The model under review builds one solid part; all positions refer to its coordinate system, in mm. Face numbers are marked on the shaded views. A direction names the side the tool comes from. Give positions to 0.01 mm unless a question says otherwise; leave off trailing zeros. Order: outer loops, then holes, each group sorted by start corner. A loop starts at its lowest first (then second) coordinate and runs counter-clockwise, first axis right, second up.
```python
from build123d import *

# Parameters (mm, degrees)
SKETCH_1_R          = 7.5
EXTRUDE_1_DEPTH     = 12.6
SKETCH_2_W          = 11.291748881
SKETCH_2_H          = 5
EXTRUDE_2_DEPTH     = 32.6
SKETCH_3_R          = 1.5
CUT_EXTRUDE_1_DEPTH = 45.373528145
FILLET_1_R          = 3
SKETCH_4_W          = 3
SKETCH_4_H          = 10
EXTRUDE_3_DEPTH     = 20
SKETCH_5_R          = 1.3
CUT_EXTRUDE_2_DEPTH = 46.967488511
SKETCH_6_W          = 35.293936169
SKETCH_6_H          = 34.958158763
CUT_EXTRUDE_3_DEPTH = 46.967488511
EXTRUDE_4_OUTLINE_R = 1.55
EXTRUDE_4_DEPTH     = 3
SKETCH_8_R          = 1.900956558
CUT_EXTRUDE_4_DEPTH = 46.967488511
SKETCH_9_R          = 3
CUT_EXTRUDE_5_DEPTH = 3


# Read off the part's stored shape, not the designer's step: 凸台-拉伸4
with BuildPart() as part:
    # 草图1 → 凸台-拉伸1 (new body)
    with BuildSketch(Plane.XY):
        with BuildLine():
            Line((-10.956194261, 6.017624724), (-22.5, -15))
            Line((-22.5, -15), (-22.5, -20))
            Line((-22.5, -20), (22.5, -20))
            Line((22.5, -20), (22.5, -15))
            Line((22.5, -15), (10.956194261, 6.017624724))
            ThreePointArc((10.956194261, 6.017624724), (0, 12.5), (-10.956194261, 6.017624724))
        make_face()
        Circle(SKETCH_1_R, mode=Mode.SUBTRACT)
    extrude(amount=EXTRUDE_1_DEPTH)

    # 草图2 → 凸台-拉伸2 (add)
    with BuildSketch(Plane.XY):
        with Locations((-16.854125559, -17.5)):
            Rectangle(SKETCH_2_W, SKETCH_2_H)
        with Locations((16.854125559, -17.5)):
            Rectangle(SKETCH_2_W, SKETCH_2_H)
    extrude(amount=EXTRUDE_2_DEPTH)

    # 草图3 → 切除-拉伸1 (cut, through all)
    with BuildSketch(Plane(origin=(0, 0, 0), x_dir=(1, 0, 0), z_dir=(0, 1, 0))):
        with Locations(Location((-17.5, -26.3, 0), (0, 0, 270))):
            Circle(SKETCH_3_R)
        with Locations((17.5, -26.3)):
            Circle(SKETCH_3_R)
    extrude(amount=-CUT_EXTRUDE_1_DEPTH, mode=Mode.SUBTRACT)

    # 圆角1
    fillet_1_edges = [part.edges().sort_by_distance(p)[0] for p in [
        (-22.5, -17.5, 32.6),
        (-11.208251119, -17.5, 32.6),
        (11.208251119, -17.5, 32.6),
    ]]
    fillet(fillet_1_edges, radius=FILLET_1_R)

    # 草图4 → 凸台-拉伸3 (add, through all)
    with BuildSketch(Plane(origin=(0, 0, 0), x_dir=(1, 0, 0), z_dir=(0, 1, 0))):
        with Locations((24, -27.6)):
            Rectangle(SKETCH_4_W, SKETCH_4_H)
    extrude(amount=-EXTRUDE_3_DEPTH)

    # 草图5 → 切除-拉伸2 (cut, through all)
    with BuildSketch(Plane(origin=(0, 0, 0), x_dir=(0, 0, -1), z_dir=(1, 0, 0))):
        with Locations(Location((-27.6, -3, 0), (0, 0, 180))):
            Circle(SKETCH_5_R)
        with Locations(Location((-27.6, -12.5, 0), (0, 0, 180))):
            Circle(SKETCH_5_R)
    extrude(amount=CUT_EXTRUDE_2_DEPTH, mode=Mode.SUBTRACT)

    # 草图6 → 切除-拉伸3 (cut, through all)
    with BuildSketch(Plane(origin=(0, 0, 0), x_dir=(0, 0, -1), z_dir=(1, 0, 0))):
        with Locations((-16.337308601, -3.7126914)):
            Rectangle(SKETCH_6_W, SKETCH_6_H)
    extrude(amount=-CUT_EXTRUDE_3_DEPTH, mode=Mode.SUBTRACT)

    # 凸台-拉伸4 outline → 凸台-拉伸4 (add)
    with BuildSketch(Plane(origin=(0, 0, 0), x_dir=(0, 0, -1), z_dir=(1, 0, 0))):
        with BuildLine():
            Line((-9.3, 15.5), (-9.3, 9.152926334))
            Line((-9.3, 9.152926334), (-3.3, 9.152926334))
            Line((-3.3, 9.152926334), (-3.3, 15.5))
            ThreePointArc((-3.3, 15.5), (-6.3, 18.5), (-9.3, 15.5))
        make_face()
        with Locations((-6.3, 15.5)):
            Circle(EXTRUDE_4_OUTLINE_R, mode=Mode.SUBTRACT)
    extrude(amount=EXTRUDE_4_DEPTH)

    # 草图8 → 切除-拉伸4 (cut, through all)
    with BuildSketch(Plane(origin=(0, 0, 0), x_dir=(0, 0, -1), z_dir=(1, 0, 0))):
        with Locations(Location((-6.3, -12.5, 0), (0, 0, 90))):
            Circle(SKETCH_8_R)
    extrude(amount=CUT_EXTRUDE_4_DEPTH, mode=Mode.SUBTRACT)

    # 草图9 → 切除-拉伸5 (cut)
    with BuildSketch(Plane(origin=(22.5, 0, 0), x_dir=(0, 0, -1), z_dir=(1, 0, 0))):
        with Locations((-6.3, -12.5)):
            Circle(SKETCH_9_R)
    extrude(amount=-CUT_EXTRUDE_5_DEPTH, mode=Mode.SUBTRACT)


solid = part.part
```
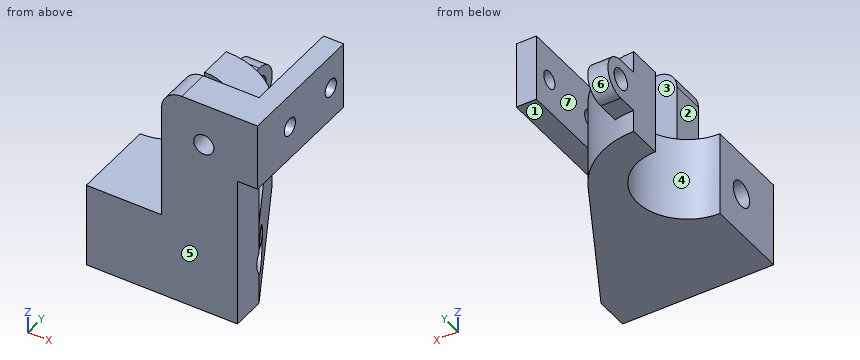
1. Take a section at A-A (x = 17.5). Write out the cut boundary in (y, z), and give its area (3 significant figures).
2. For the marked faces 1, 2 and 3, list the 3-axis set-ups (+Z, -Z, +X, -X, +Y, -Y) from which the entire face can be reached by the end or side of a thin tool; tool diameter is ignored.
3. Insertion check: pin 1 (9.5 mm diameter, centred on y = -12.5, z = 6.3, fed in from +X); pin 2 (3.5 mm diameter, centred on x = 18.5, z = 23, fed in from +Y); pin 3 (1.5 mm diameter, centred on x = 1.5, y = 13.5, fed in from +Z); pin 4 (3 mm diameter, centred on y = -12.5, z = 6.3, fed in from +X). Each pin has a flat end and moves straight along its axis. Give the tip position at first contact, or say it passes through.
4. Take a section at C-C (z = 24). Write out the cut boundary in (x, y), and give its area (3 significant figures).
5. Draft analysis for pull direction Y (two halves, no side actions). For the marked faces 4, 5, 6 and 7, state which applies: pulls with the +Y half, pulls with the -Y half, needs draft (parallel to the pull), parting line crosses it, or undercut.
6. Take a section at B-B (y = -12.5). Write out the cut boundary in (x, z).
7. To check wall thickness, follow line 1 (Y direction, x = 23.75, z = 27.6); line 2 (Y direction, x = 5.5, z = 6.3); line 3 (X direction, y = -18.2, z = 26.3). State the ranges of each line that lie inside material, in increasing order.
8. Take a section at D-D (x = 12). Write out the cut boundary in (y, z).
Answer:
1. outline: (-20, 0) - (-5.9, 0) - (-5.9, 12.6) - (-15, 12.6) - (-15, 24.8) - (-20, 24.8) - close; (-20, 27.8) - (-15, 27.8) - (-15, 32.6) - (-20, 32.6) - close; hole circle Ø3.8 at (-12.5, 6.3)
1. area: 251 mm2
2. face 1: -Z, +X, +Y, -Y
2. face 2: +Z, -X, +Y, -Y
2. face 3: +Z, -X, +Y
3. pin 1: stops at x = 22.5
3. pin 2: stops at y = -15
3. pin 3: stops at z = 9.3
3. pin 4: passes through
4. outline: (11.21, -20) - (25.5, -20) - (25.5, 0) - (22.5, 0) - (22.5, -15) - (11.21, -15) - close
4. area: 116 mm2
5. face 4: undercut
5. face 5: pulls with the -Y half
5. face 6: pulls with the +Y half
5. face 7: needs draft
6. outline: (0, 0) - (21.13, 0) - (21.13, 3.3) - (19.5, 3.3) - (19.5, 4.4) - (0, 4.4) - close; (0, 8.2) - (19.5, 8.2) - (19.5, 9.3) - (21.13, 9.3) - (21.13, 12.6) - (0, 12.6) - close; (22.5, 22.6) - (25.5, 22.6) - (25.5, 26.3) - (22.5, 26.3) - close; (22.5, 28.9) - (25.5, 28.9) - (25.5, 32.6) - (22.5, 32.6) - close
7. line 1: y = -20 to -13.8, -11.2 to -4.3, -1.7 to 0
7. line 2: y = -20 to -14.4, -10.6 to -5.1, 5.1 to 11.22
7. line 3: x = 11.21 to 16, 19 to 25.5
8. outline: (-20, 0) - (4.12, 0) - (4.12, 12.6) - (-15, 12.6) - (-15, 31.63) - (-20, 31.63) - close; hole circle Ø3.8 at (-12.5, 6.3)
